Geometry check sheet. Reference: the model listing, model coordinates, mm. Face numbers are marked on the shaded views. A direction names the side the tool comes from. Coordinates: 2 decimals unless noted, no trailing zeros. Write each loop counter-clockwise with the first axis right and the second up, starting at its lowest first coordinate (ties: lowest second). Pieces come first, ordered by that corner, then holes. Notation, with made-up numbers: (86, 70.25) -> (98, 70.25) arc R19 ccw to (98, 83.25) -> close; hole circle Ø9 at (34, -9). An arc over 180 degrees is marked (long way). Answer as CSV lines item,"result".
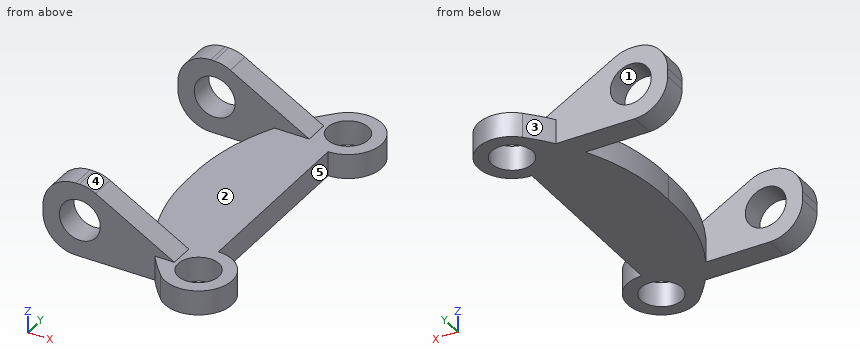
```python
from build123d import *

# Parameters (mm, degrees)
CROQUIS2_R              = 2.5
SALIENTE_EXTRUIR1_DEPTH = 3
SALIENTE_EXTRUIR2_START = 12.5
CROQUIS4_R              = 2.5
SALIENTE_EXTRUIR2_DEPTH = 3


with BuildPart() as part:
    # Croquis2 → Saliente-Extruir1 (new body)
    with BuildSketch(Plane.XY):
        with BuildLine():
            Line((3.492952335, 10.790611409), (3.492952335, -11.964892683))
            ThreePointArc((3.492952335, -11.964892683), (7.2895288, -17.69304703), (0.534883591, -18.958160926))
            ThreePointArc((0.534883591, -18.958160926), (-4.86923602, -10.494496462), (-6.507047205, -0.587140637))
            ThreePointArc((-6.507047205, -0.587140637), (-4.86923602, 9.320215188), (0.534883591, 17.783879652))
            ThreePointArc((0.534883591, 17.783879652), (7.2895288, 16.518765755), (3.492952335, 10.790611409))
        make_face()
        with Locations((3.492952335, 14.912859363)):
            Circle(CROQUIS2_R, mode=Mode.SUBTRACT)
        with Locations((3.492952335, -16.087140637)):
            Circle(CROQUIS2_R, mode=Mode.SUBTRACT)
    extrude(amount=SALIENTE_EXTRUIR1_DEPTH)

    # Croquis4 → Saliente-Extruir2 (add)
    with BuildSketch(Plane(origin=(0, -0.587140637, 0), x_dir=(1, 0, 0), z_dir=(0, 1, 0)).offset(SALIENTE_EXTRUIR2_START)):
        with BuildLine():
            Line((0.534883591, -3), (-9.106451157, -8.477853714))
            ThreePointArc((-9.106451157, -8.477853714), (-10.060534072, -8.867260972), (-11.082440414, -9))
            Line((-11.082440414, -9), (-11.52545838, -9))
            ThreePointArc((-11.52545838, -9), (-14.353885504, -7.828427125), (-15.52545838, -5))
            Line((-15.52545838, -5), (-15.52545838, -4))
            ThreePointArc((-15.52545838, -4), (-14.353885504, -1.171572875), (-11.52545838, 0))
            Line((-11.52545838, 0), (0.534883591, 0))
            Line((0.534883591, 0), (0.534883591, -3))
        make_face()
        with Locations(Location((-11.02545838, -4.5, 0), (0, 0, 180))):
            Circle(CROQUIS4_R, mode=Mode.SUBTRACT)
    saliente_extruir2 = extrude(amount=SALIENTE_EXTRUIR2_DEPTH)

    # Simetría1: Saliente-Extruir2 across plane
    add(saliente_extruir2.mirror(Plane.ZX.offset(-0.587140637)))


solid = part.part
```
Item 1: Depth check by flat-ended pin: pin 1 Ø4 at (x, y) = (3.49, 14.91) entering from -Z; pin 2 Ø1.5 at (y, z) = (-3, 2) entering from +X; pin 3 Ø1.5 at (x, y) = (-4.5, -2) entering from +Z; pin 4 Ø2.5 at (x, z) = (-4, 6) entering from -Y. Enter the tip coordinate at first touch or a pass-through.
Responses:
pin 1,"passes through"
pin 2,"stops at x = 3.49"
pin 3,"stops at z = 3"
pin 4,"stops at y = -16.09"
Item 2: Set-up check for the marked faces 4 and 5: record each of +Z, -Z, +X, -X, +Y, -Y from which the full face is reachable in a straight line by a thin tool's end or side.
Responses:
face 4,"+Z, +X, +Y, -Y"
face 5,"+Z, -Z, +X"
Item 3: Cross-section at B-B, the plane x = -8. Record the cut outline in (y, z).
Responses:
outline,"(-16.09, 0) -> (-13.09, 0) -> (-13.09, 7.85) -> (-16.09, 7.85) -> close; (11.91, 0) -> (14.91, 0) -> (14.91, 7.85) -> (11.91, 7.85) -> close"
Item 4: Cross-section at D-D, the plane y = -2.5. Record the cut outline in (x, z), plus the area to 3 significant figures.
Responses:
outline,"(-6.51, 0) -> (3.49, 0) -> (3.49, 3) -> (-6.51, 3) -> close"
area,"30.0 mm2"
Item 5: Release check for a two-part mould opening along Z. For the marked faces 1, 2 and 3 record: +Z half, -Z half, draft (parallel to the pull), parting line (faces both ways), or undercut.
Responses:
face 1,"undercut"
face 2,"+Z half"
face 3,"draft"
Item 6: Cross-section at A-A, the plane z = 7.5. Record the cut outline in (x, y), plus the area to 3 significant figures.
Responses:
outline,"(-14.65, -16.09) -> (-7.39, -16.09) -> (-7.39, -13.09) -> (-14.65, -13.09) -> close; (-14.65, 11.91) -> (-7.39, 11.91) -> (-7.39, 14.91) -> (-14.65, 14.91) -> close"
area,"43.6 mm2"
Item 7: Cross-section at C-C, the plane z = 4.5. Record the cut outline in (x, y), plus the area to 3 significant figures.
Responses:
outline,"(-15.53, -16.09) -> (-13.53, -16.09) -> (-13.53, -13.09) -> (-15.53, -13.09) -> close; (-15.53, 11.91) -> (-13.53, 11.91) -> (-13.53, 14.91) -> (-15.53, 14.91) -> close; (-8.53, -16.09) -> (-2.11, -16.09) -> (-2.11, -13.09) -> (-8.53, -13.09) -> close; (-8.53, 11.91) -> (-2.11, 11.91) -> (-2.11, 14.91) -> (-8.53, 14.91) -> close"
area,"50.5 mm2"
Item 8: Thickness scan on probe 1 along Y at (x, z) = (-10.25, 7.5); probe 2 along Y at (x, z) = (3.75, 1); probe 3 along Z at (x, y) = (0, 10). Record the ranges inside material, lowest first.
Responses:
probe 1,"y = -16.09 to -13.09, 11.91 to 14.91"
probe 2,"y = -20.2 to -18.57, -13.6 to -11.97, 10.8 to 12.43, 17.4 to 19.03"
probe 3,"z = 0 to 3"
